Can you work these out from the model? Positions are in its coordinate system, mm. A direction names the side the tool comes from. Give positions to 0.01 mm unless a question says otherwise; leave off trailing zeros. Order: outer loops, then holes, each group sorted by start corner. A loop starts at its lowest first (then second) coordinate and runs counter-clockwise, first axis right, second up. Notation, with made-up numbers: M 86.5,-31 L 112.5,-31 A26 cw 112.5,3 Z; hole C 64,76 d4. An arc over 180 degrees is marked long. Use a Markdown table: item, result. Add a question column.
from build123d import *

# Parameters (mm, degrees)
SKETCH1_W           = 550
SKETCH1_H           = 550
BOSS_EXTRUDE1_DEPTH = 50
SKETCH2_W           = 500
SKETCH2_H           = 500
CUT_EXTRUDE1_DEPTH  = 40
BOSS_EXTRUDE2_DEPTH = 34
CIRPATTERN1_COUNT   = 4


with BuildPart() as part:
    # Sketch1 → Boss-Extrude1 (new body)
    with BuildSketch(Plane(origin=(0, 0, 0), x_dir=(1, 0, 0), z_dir=(0, 1, 0))):
        Rectangle(SKETCH1_W, SKETCH1_H)
    extrude(amount=BOSS_EXTRUDE1_DEPTH)

    # Sketch2 → Cut-Extrude1 (cut)
    with BuildSketch(Plane(origin=(0, 50, 0), x_dir=(1, 0, 0), z_dir=(0, 1, 0))):
        Rectangle(SKETCH2_W, SKETCH2_H)
    extrude(amount=-CUT_EXTRUDE1_DEPTH, mode=Mode.SUBTRACT)

    # Sketch3 → Boss-Extrude2 (add)
    with BuildSketch(Plane(origin=(0, 10, 0), x_dir=(1, 0, 0), z_dir=(0, 1, 0))):
        Polygon((-250, 250), (-220, 250), (-250, 220), align=None)
    boss_extrude2 = extrude(amount=BOSS_EXTRUDE2_DEPTH)

    # CirPattern1: Boss-Extrude2 ×4 about axis
    cirpattern1_axis = Axis((0.432779002, 0, 0.432779002), (0, 1, 0))
    for i in range(1, CIRPATTERN1_COUNT):
        add(boss_extrude2.rotate(cirpattern1_axis, i * 360 / CIRPATTERN1_COUNT))


solid = part.part
1. I need wall thicknesses on L1, parallel to X at y = 20, z = 135.5; L2, parallel to Y at x = -230, z = 247. Which ranges of each line are inside material? Lowest first, please. Write a range as [from, to].
2. If we section it at C-C, the plane y = 26.5: List the corners of the cut face in (x, z) for me, then the cut area to 3 significant figures.
3. On a 3-axis mill with a long thin cutter (end or side, diameter ignored), from which of +Z, -Z, +X, -X, +Y, -Y can I reach the whole of each face in a straight line? I mean faces 1 (the face through (-22, 50, 264)), 2 (the face through (-235, 27, -235)). Say none if no direction works.
4. We'd pull the mould along Z, two halves only. Please class faces 3 (the face through (-275, 25, 4)), 4 (the face through (250, 30, 3)), 5 (the face through (-4, 25, -275)): +Z half, -Z half, draft (parallel to the pull), parting line (faces both ways), or undercut.
5. If we section it at B-B, the plane x = -15: List the corners of the cut face in (y, z) for me.
6. If we section it at D-D, the plane z = 230: List the corners of the cut face in (x, y) for me.
7. Will these pins go through, and if not, where does the flat tip stop? pin 1 (1.5 mm diameter, centred on x = -119.5, z = 5, fed in from -Y); pin 2 (14.5 mm diameter, centred on x = 230, z = -241, fed in from +Y); pin 3 (2 mm diameter, centred on x = 5.5, z = 176.5, fed in from +Y).
8. If we section it at A-A, the plane z = -37: List the corners of the cut face in (x, y) for me, then the cut area to 3 significant figures.
Geometry results:
| question | item | result |
|---|---|---|
| 1 | L1 | x = [-275, -250], [250, 275] |
| 1 | L2 | y = [0, 44] |
| 2 | outline | M -275,-275 L 275,-275 L 275,275 L -275,275 Z; hole M -250,-220 L -220,-250 L 220.87,-250 L 250,-220.87 L 250,221.73 L 221.73,250 L -220.87,250 L -250,220.87 Z |
| 2 | area | 54,200 mm^2 |
| 3 | face 1 | +Z, -Z, +X, -X, +Y |
| 3 | face 2 | +Y |
| 4 | face 3 | draft |
| 4 | face 4 | undercut |
| 4 | face 5 | -Z half |
| 5 | outline | M 0,-275 L 50,-275 L 50,-250 L 10,-250 L 10,250 L 50,250 L 50,275 L 0,275 Z |
| 6 | outline | M -275,0 L 275,0 L 275,50 L 250,50 L 250,44 L 241.73,44 L 241.73,10 L -240.87,10 L -240.87,44 L -250,44 L -250,50 L -275,50 Z |
| 7 | pin 1 | stops at y = 0 |
| 7 | pin 2 | stops at y = 44 |
| 7 | pin 3 | stops at y = 10 |
| 8 | outline | M -275,0 L 275,0 L 275,50 L 250,50 L 250,10 L -250,10 L -250,50 L -275,50 Z |
| 8 | area | 7,500 mm^2 |
